from build123d import *

# Parameters (mm, degrees)
SKETCH_1_W          = 40
SKETCH_1_H          = 25
EXTRUDE_1_DEPTH     = 30
SKETCH_2_W          = 40
SKETCH_2_H          = 2
CUT_EXTRUDE_1_DEPTH = 24
SKETCH_3_W          = 2
SKETCH_3_H          = 25
CUT_EXTRUDE_2_DEPTH = 24
SKETCH_4_R          = 1
CUT_EXTRUDE_3_DEPTH = 3


with BuildPart() as part:
    # 草图1 → 拉伸1 (new body)
    with BuildSketch(Plane(origin=(0, 0, 0), x_dir=(1, 0, 0), z_dir=(0, 1, 0))):
        Rectangle(SKETCH_1_W, SKETCH_1_H)
    extrude(amount=EXTRUDE_1_DEPTH)

    # 草图2 → 切除-拉伸1 (cut)
    with BuildSketch(Plane(origin=(0, 30, 0), x_dir=(-1, 0, 0), z_dir=(0, 1, 0))):
        with Locations((0, -10.5)):
            Rectangle(SKETCH_2_W, SKETCH_2_H)
        with Locations((0, -6.25)):
            Rectangle(SKETCH_2_W, SKETCH_2_H)
        with Locations((0, -2)):
            Rectangle(SKETCH_2_W, SKETCH_2_H)
        with Locations((0, 2.25)):
            Rectangle(SKETCH_2_W, SKETCH_2_H)
        with Locations((0, 6.5)):
            Rectangle(SKETCH_2_W, SKETCH_2_H)
        with Locations((0, 10.75)):
            Rectangle(SKETCH_2_W, SKETCH_2_H)
    extrude(amount=-CUT_EXTRUDE_1_DEPTH, mode=Mode.SUBTRACT)

    # 草图3 → 切除-拉伸2 (cut)
    with BuildSketch(Plane(origin=(0, 30, 0), x_dir=(-1, 0, 0), z_dir=(0, 1, 0))):
        with Locations((-7, 0)):
            Rectangle(SKETCH_3_W, SKETCH_3_H)
        with Locations((9.5, 0)):
            Rectangle(SKETCH_3_W, SKETCH_3_H)
    extrude(amount=-CUT_EXTRUDE_2_DEPTH, mode=Mode.SUBTRACT)

    # 草图4 → 切除-拉伸3 (cut)
    with BuildSketch(Plane.XZ):
        with Locations(Location((16, 0, 0), (0, 0, 270))):
            Circle(SKETCH_4_R)
        with Locations(Location((-16, 0, 0), (0, 0, 90))):
            Circle(SKETCH_4_R)
    extrude(amount=-CUT_EXTRUDE_3_DEPTH, mode=Mode.SUBTRACT)


solid = part.part
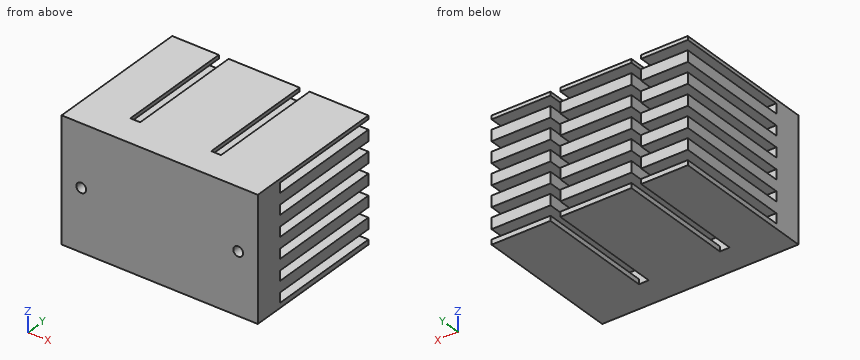
Source: CAD feature listing. Evaluate the final solid. Frame: model axes, mm. Coordinates: 2 decimals unless noted, no trailing zeros. Order: outer loops, then holes, each group sorted by start corner. A loop starts at its lowest first (then second) coordinate and runs counter-clockwise, first axis right, second up. Notation, with made-up numbers: M 53,6.5 L 94,6.5 A13 cw 94,19.5 Z; hole C 29.5,-19.75 d7. An arc over 180 degrees is marked long. Write each question's results on one line, items separated by ' | '. Start each with the question number.
Item 1: Cut plane B-B (z = 0). Return loops of the section in (x, y), and give its area (3 significant figures).
Item 2: Cut plane C-C (y = 11.75). Count the separate pieces of the cut face and the enclosed holes in it, and give its area (3 significant figures).
Item 3: Line query: probe 1 along X at (y, z) = (20.75, -0.75); probe 2 along X at (y, z) = (1.6, 0); probe 3 along Z at (x, y) = (-16, 1.35). Output: solid intervals per line, ascending.
Item 4: Cut plane A-A (x = -5). Return loops of the section in (y, z).
Item 5: First-contact query: pin 1 Ø5 at (x, z) = (2.5, -2.5) entering from +Y. Flat tip, straight axial feed; report the tip coordinate or a pass-through.
Checked values:
1) outline: M -20,0 L -17,0 L -17,3 L -15,3 L -15,0 L 15,0 L 15,3 L 17,3 L 17,0 L 20,0 L 20,30 L 8,30 L 8,6 L 6,6 L 6,30 L -8.5,30 L -8.5,6 L -10.5,6 L -10.5,30 L -20,30 Z | area: 1,090 mm2
2) separate pieces: 21 | enclosed holes: 0 | area: 468 mm2
3) probe 1: x = -20 to -10.5, -8.5 to 6, 8 to 20 | probe 2: x = -20 to -17, -15 to 15, 17 to 20 | probe 3: z = -12.5 to -1, 1 to 12.5
4) outline: M 0,-12.5 L 30,-12.5 L 30,-11.5 L 6,-11.5 L 6,-9.5 L 30,-9.5 L 30,-7.25 L 6,-7.25 L 6,-5.25 L 30,-5.25 L 30,-3 L 6,-3 L 6,-1 L 30,-1 L 30,1.25 L 6,1.25 L 6,3.25 L 30,3.25 L 30,5.5 L 6,5.5 L 6,7.5 L 30,7.5 L 30,9.75 L 6,9.75 L 6,11.75 L 30,11.75 L 30,12.5 L 0,12.5 Z
5) pin 1: stops at y = 30
